```python
from build123d import *

# Parameters (mm, degrees)
F2_SIZE = 2


with BuildPart() as f1:
    # F0 (on Front) → F1 (revolve)
    with BuildSketch(Plane.XZ):
        with BuildLine():
            Line((20.5, 50), (0, 50))
            Line((0, 50), (0, 0))
            Line((0, 0), (45, 0))
            Line((45, 0), (45, 18))
            ThreePointArc((45, 18), (44.414214, 19.414214), (43, 20))
            Line((43, 20), (38.333333, 20))
            ThreePointArc((38.333333, 20), (35.559832, 20.839749), (33.717949, 23.076923))
            Line((33.717949, 23.076923), (23.269231, 48.153846))
            ThreePointArc((23.269231, 48.153846), (22.164101, 49.496151), (20.5, 50))
        make_face()
    revolve(axis=Axis((0, 0, 16.569998), (0, 0, 1)))

    # F2
    f2_edges = [f1.edges().sort_by_distance(p)[0] for p in [
        (-45, 0, 0),
    ]]
    chamfer(f2_edges, length=F2_SIZE)


solid = f1.part
```
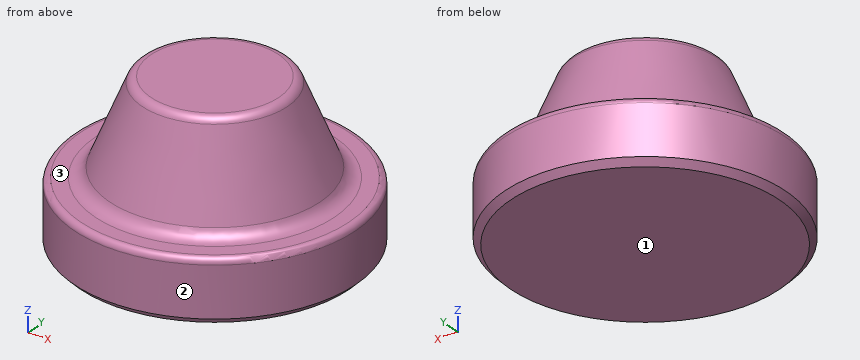
For this review, take the finished solid that the model builds, in its own axes (mm). Face numbers are marked on the shaded views. Coordinates: 2 decimals unless noted, no trailing zeros. Write each loop counter-clockwise with the first axis right and the second up, starting at its lowest first coordinate (ties: lowest second). Pieces come first, ordered by that corner, then holes.
(1) Add section A-A on y = 0. Give the boundary of the cut face in (x, z).
(2) The part is to be moulded in two halves that separate along Z. For the marked faces 1, 2 and 3, say which applies: +Z half, -Z half, draft (parallel to the pull), parting line (faces both ways), or undercut.
(3) Add section D-D on z = 28. Give the boundary of the cut face in (x, y), then the cut area to 3 significant figures.
(4) For pin 1 Ø1.5 at (x, z) = (-2.5, 24.5) entering from +Y; pin 2 Ø1 at (x, z) = (-6, 21.5) entering from -Y; pin 3 Ø1 at (y, z) = (-34, 25.5) entering from +X; pin 4 Ø5 at (y, z) = (20.5, 9.5) entering from +X, all flat-tipped, find the tip position at first contact; note any pin that passes through.
(5) Add section C-C on z = 15.5. Give the boundary of the cut face in (x, y), then the cut area to 3 significant figures.
(6) Wall thickness on probe 1 along Z at (x, y) = (14.5, -40.5); probe 2 along X at (y, z) = (1, 16); probe 3 along Y at (x, z) = (-12, 43.5): over which ranges is each line inside the solid? List them lowest first.
Answer sheet:
1. outline: (-45, 2) - (-43, 0) - (43, 0) - (45, 2) - (45, 18) arc R2 ccw to (43, 20) - (38.33, 20) arc R5 cw to (33.72, 23.08) - (23.27, 48.15) arc R3 ccw to (20.5, 50) - (-20.5, 50) arc R3 ccw to (-23.27, 48.15) - (-33.72, 23.08) arc R5 cw to (-38.33, 20) - (-43, 20) arc R2 ccw to (-45, 18) - close
2. face 1: -Z half
2. face 2: draft
2. face 3: +Z half
3. outline: circle Ø63.33 at (0, 0)
3. area: 3,150 mm2
4. pin 1: stops at y = 33.35
4. pin 2: stops at y = -34.83
4. pin 3: passes through
4. pin 4: stops at x = 41.24
5. outline: circle Ø90 at (0, 0)
5. area: 6,360 mm2
6. probe 1: z = 0.02 to 20
6. probe 2: x = -44.99 to 44.99
6. probe 3: y = -22.17 to 22.17
